from build123d import *

# Parameters (mm, degrees)
F0_R     = 31.75
F1_DEPTH = 19.05
F2_W     = 101.6
F2_H     = 19.05
F3_DEPTH = 50.8
F4_W     = 19.05
F4_H     = 19.05
F5_DEPTH = 19.05


with BuildPart() as f1:
    # F0 (on Top) → F1 (new body)
    with BuildSketch(Plane.XY):
        with BuildLine():
            ThreePointArc((50.8, 12.7), (35.921024, 48.621024), (0, 63.5))
            ThreePointArc((0, 63.5), (-35.921024, 48.621024), (-50.8, 12.7))
            Line((-50.8, 12.7), (-50.8, -63.5))
            Line((-50.8, -63.5), (50.8, -63.5))
            Line((50.8, -63.5), (50.8, 12.7))
        make_face()
        with Locations((0, 12.7)):
            Circle(F0_R, mode=Mode.SUBTRACT)
    extrude(amount=F1_DEPTH)

    # F2 (on face) → F3 (join)
    with BuildSketch(Plane.XY.offset(19.05)):
        with Locations((0, -53.975)):
            Rectangle(F2_W, F2_H)
    extrude(amount=F3_DEPTH)

    # F4 (on face) → F5 (cut)
    with BuildSketch(Plane.XY.offset(69.85)):
        with Locations((41.275, -53.975)):
            Rectangle(F4_W, F4_H)
    extrude(amount=-F5_DEPTH, mode=Mode.SUBTRACT)


solid = f1.part
Read the model definition and answer for the solid it produces. Units are mm, in the model's axes. A direction names the side the tool comes from. Coordinates: 2 decimals unless noted, no trailing zeros. Loops run counter-clockwise (first coordinate to the right, second up) from the corner with the lowest first, then second, coordinate; pieces in that order, holes last.
Q1. The part is cut by section A-A on x = 13.5. Write down the section's boundary in (y, z).
Q2. Each of these flat-tipped pins is pushed along its axis until it touches: pin 1 Ø21 at (y, z) = (-54.5, 62.5) entering from +X; pin 2 Ø3 at (x, z) = (-5.5, 53.5) entering from +Y; pin 3 Ø5 at (x, y) = (4.5, 44.5) entering from +Z. Where does it stop, or does it pass through?
Q3. Consider probe 1 along Y at (x, z) = (0, 6); probe 2 along X at (y, z) = (12, 5); probe 3 along Z at (x, y) = (-39.5, 42). Determine where each line is inside the solid, lowest interval first.
Q4. Which of the six approach directions +Z, -Z, +X, -X, +Y, -Y give full straight-line access (tool end or side, diameter ignored) to faces 5 (the face through (22, -14, 19.05)), 6 (the face through (41, -54, 50.8)), 7 (the face through (50.8, -34, 14))?
Q5. The part is cut by section B-B on y = 34.5. Write down the section's boundary in (x, z).
Q6. The mould has two halves that part along X. Classify faces 1 (the face through (-6.883, -18.295, 9.392)), 2 (the face through (-50.8, -34.4, 18.9)), 3 (the face through (-1, -44.45, 44)), 4 (the face through (31.75, -54, 60)): +X half, -X half, draft (parallel to the pull), parting line (faces both ways), or undercut.
Q7. The part is cut by section D-D on x = 39.5. Write down the section's boundary in (y, z).
Q8. The part is cut by section C-C on z = 4.5. Write down the section's boundary in (x, y), and give its area (3 significant figures).
Results below:
1. outline: (-63.5, 0) - (-16.04, 0) - (-16.04, 19.05) - (-44.45, 19.05) - (-44.45, 69.85) - (-63.5, 69.85) - close; (41.44, 0) - (61.67, 0) - (61.67, 19.05) - (41.44, 19.05) - close
2. pin 1: stops at x = 31.75
2. pin 2: stops at y = -44.45
2. pin 3: stops at z = 19.05
3. probe 1: y = -63.5 to -19.05, 44.45 to 63.5
3. probe 2: x = -50.8 to -31.74, 31.74 to 50.8
3. probe 3: z = 0 to 19.05
4. face 5: +Z, +X, -X, +Y
4. face 6: +Z, +X, +Y, -Y
4. face 7: +Z, -Z, +X, +Y, -Y
5. outline: (-45.88, 0) - (-23.08, 0) - (-23.08, 19.05) - (-45.88, 19.05) - close; (23.08, 0) - (45.88, 0) - (45.88, 19.05) - (23.08, 19.05) - close
6. face 1: undercut
6. face 2: -X half
6. face 3: draft
6. face 4: +X half
7. outline: (-63.5, 0) - (44.64, 0) - (44.64, 19.05) - (-44.45, 19.05) - (-44.45, 50.8) - (-63.5, 50.8) - close
8. outline: (-50.8, -63.5) - (50.8, -63.5) - (50.8, 12.7) arc R50.8 ccw to (0, 63.5) arc R50.8 ccw to (-50.8, 12.7) - close; hole circle Ø63.5 at (0, 12.7)
8. area: 8,630 mm2
